Geometry check sheet. Reference: the model listing, model coordinates, mm. A direction names the side the tool comes from. Round coordinates to 2 decimals unless told otherwise and drop trailing zeros. Order: outer loops, then holes, each group sorted by start corner. A loop starts at its lowest first (then second) coordinate and runs counter-clockwise, first axis right, second up.
(1) Cross-section at A-A on x = 19. Enter the section's corners in (y, z).
(2) Gauge pin test, flat ends, axial feed: P1, Ø4, axis at x = -3.5, z = 2.5, coming from the +Y side; P2, Ø5.5, axis at x = 0, z = 0, coming from the -Y side; P3, Ø1, axis at x = 5.5, y = 20, coming from the +Z side. Record the tip position at first contact, or that the pin passes through.
(3) Cross-section at C-C on y = 2.5. Enter the section's corners in (x, z), and give its area (3 significant figures).
(4) Draft check along Z on faces 4 (the face through (-2.23, -15.93, 2.43)), 5 (the face through (0, -14, 10)), 6 (the face through (13.3, 16, 0.1)), 7 (the face through (0, -11, 5)). Enter one of: pulls with the +Z half, pulls with the -Z half, needs draft (parallel to the pull), parting line crosses it, or undercut.
(5) Thickness scan on L1, parallel to X at y = -16.75, z = 0; L2, parallel to Y at x = -0.5, z = 9; L3, parallel to X at y = -2, z = 1. Record the ranges inside material, lowest first.
(6) Cross-section at B-B on z = -7.5. Enter the section's corners in (x, y), and give its area (3 significant figures).
(7) Set-up check for faces 1 (the face through (0, 19, 5)), 2 (the face through (23.6, 12.14, -0.14)), 3 (the face through (-9.28, -15.93, 0.72)): record each of +Z, -Z, +X, -X, +Y, -Y from which the full face is reachable in a straight line by a thin tool's end or side.
(8) Cross-section at D-D on y = 17. Enter the section's corners in (x, z).
Autodesk Inventor part; units mm, degrees
ref_plane "Work Plane1" through (-32.5, 0, 0) normal (1, 0, 0) x (0, 1, 0)
ref_plane "XZ Plane" through (0, 0, 0) normal (0, 1, 0) x (-1, 0, 0)
ref_plane "XY Plane" through (0, 0, 0) normal (0, 0, 1) x (1, 0, 0)
ref_plane "Work Plane1" through (-32.5, 0, 0) normal (1, 0, 0) x (0, 1, 0)
sketch "Sketch1" plane through (-32.5, 0, 0) normal (1, 0, 0) x (0, 1, 0)
  line L0 (-21, 10) -> (-21, -10)
  line L1 (19, -3.75) -> (21, -3.75)
  line L2 (21, -10) -> (-21, -10)
  line L3 (19, 10) -> (19, -3.75)
  line L4 (19, 10) -> (-21, 10)
  line L5 (21, -3.75) -> (21, -10)
extrude "Extrusion4" add sketch "Sketch1" along normal blind 65
sketch "Sketch2" plane through (-32.5, -21, 10) normal (0, 0, 1) x (1, 0, 0)
  line L0 (57, 10) -> (57, 34)
  line L1 (57, 34) -> (8, 34)
  line L2 (8, 34) -> (8, 10)
  line L3 (8, 10) -> (57, 10)
extrude "Extrusion3" cut sketch "Sketch2" against normal blind 20
sketch "Sketch3" plane through (-32.5, 19, 10) normal (0, 1, 0) x (1, 0, 0)
  line L0 (42.5, 13.3) -> (22.5, 13.3)
  arc A0 (22.5, 13.3) -> (22.5, 6.7) centre (22.5, 10) ccw
  arc A1 (42.5, 6.7) -> (42.5, 13.3) centre (42.5, 10) ccw
  line L1 (22.5, 6.7) -> (42.5, 6.7)
extrude "Extrusion2" cut sketch "Sketch3" against normal blind 6
fillet "Fillet4" radius 3 1 edges at (24.5, 13, 0)
fillet "Fillet3" radius 3 1 edges at (24.5, -11, 0)
fillet "Fillet2" radius 3 1 edges at (-24.5, -11, 0)
fillet "Fillet1" radius 3 1 edges at (-24.5, 13, 0)
sketch "Sketch7" plane through (-32.5, -21, -10) normal (0, -1, 0) x (1, 0, 0)
  line L0 (45, 10) -> (20, 10)
  line L1 (11, 20) -> (54, 20) construction
  line L2 (32.5, 20) -> (32.5, 0) construction
  line L3 (0, 0) -> (65, 0) construction
  point P0 (32.5, 10)
  point P1 (32.5, 10)
  dimension "d41" = 25
hole "M6CLR" at (0, -21, 0) at (-12.5, -21, 0) at (12.5, -21, 0) direction (0, 1, 0) diameter 6.6 depth 10
sketch "Sketch5" plane through (-32.5, -21, -10) normal (0, -1, 0) x (1, 0, 0)
  point P0 (7.5, 10)
hole "4H7" at (-25, -21, 0) direction (0, 1, 0) diameter 4 depth 9 tip angle 118
sketch "Sketch4" plane through (-32.5, -21, -10) normal (0, -1, 0) x (1, 0, 0)
  arc A0 (60, 8) -> (60, 12) centre (60, 10) ccw
  line L0 (55, 8) -> (60, 8)
  line L1 (60, 12) -> (55, 12)
  arc A1 (55, 12) -> (55, 8) centre (55, 10) ccw
  dimension "d42" = 4
  dimension "d43" = 5
extrude "Extrusion1" cut sketch "Sketch4" against normal blind 9
properties part number "ASF-10003"
Found:
1. outline: (-21, -10) - (-11, -10) - (-11, 10) - (-21, 10) - close; (13, -10) - (21, -10) - (21, -3.75) - (19, -3.75) - (19, 10) - (13, 10) - close
2. P1: stops at y = 19
2. P2: passes through
2. P3: stops at z = -3.75
3. outline: (-32.5, -10) - (-24.5, -10) - (-24.5, 10) - (-32.5, 10) - close; (24.5, -10) - (32.5, -10) - (32.5, 10) - (24.5, 10) - close
3. area: 320 mm2
4. face 4: undercut
4. face 5: pulls with the +Z half
4. face 6: undercut
4. face 7: needs draft
5. L1: x = -32.5 to -27, -23 to -15.8, -9.2 to -3.3, 3.3 to 9.2, 15.8 to 20.5, 29.5 to 32.5
5. L2: y = -21 to -11, 13 to 19
5. L3: x = -32.5 to -24.5, 24.5 to 32.5
6. outline: (-32.5, -21) - (32.5, -21) - (32.5, 21) - (-32.5, 21) - close; hole (-24.5, -8) arc R3 ccw to (-21.5, -11) - (21.5, -11) arc R3 ccw to (24.5, -8) - (24.5, 10) arc R3 ccw to (21.5, 13) - (-21.5, 13) arc R3 ccw to (-24.5, 10) - close
6. area: 1,560 mm2
7. face 1: +Z, +X, -X, +Y
7. face 2: +Z, -Z
7. face 3: -Y
8. outline: (-32.5, -10) - (32.5, -10) - (32.5, 10) - (-32.5, 10) - close; hole (-10, -3.3) - (10, -3.3) arc R3.3 ccw to (10, 3.3) - (-10, 3.3) arc R3.3 ccw to start
